The model under review builds one solid part; all positions refer to its coordinate system, in mm. Face numbers are marked on the shaded views. A direction names the side the tool comes from. Round coordinates to 2 decimals unless told otherwise and drop trailing zeros. Write each loop counter-clockwise with the first axis right and the second up, starting at its lowest first coordinate (ties: lowest second). Pieces come first, ordered by that corner, then holes. Notation, with made-up numbers: M -22.75,88 L 7.25,88 A31 ccw 7.25,117 Z; hole C 40,41.5 d6. An arc over 180 degrees is marked long. Write item = value, one per line. Start each with the question number.
Item 1: To check wall thickness, follow line 1 along Y through (x, z) = (19, 0.25); line 2 along Z through (x, y) = (-4, -1.5); line 3 along Y through (x, z) = (-6, -0.25). State the ranges of each line that lie inside material, in increasing order.
Item 2: Take a section at D-D, the plane y = -0.5. Give the boundary of the cut face in (x, z), plus the area to 3 significant figures.
Item 3: Take a section at C-C, the plane x = -2.5. Give the boundary of the cut face in (y, z).
Item 4: Take a section at A-A, the plane x = 43. Give the boundary of the cut face in (y, z).
Item 5: For pin 1 Ø2.5 at (y, z) = (-0.5, -1.5) entering from -X; pin 2 Ø3 at (y, z) = (0, -2) entering from +X; pin 3 Ø6 at (x, y) = (39.5, 0) entering from -Z; pin 4 Ø1.5 at (x, z) = (33, -0.5) entering from -Y, all flat-tipped, find the tip position at first contact; note any pin that passes through.
Item 6: Tool access review of the marked faces 1, 2 and 3: name each direction out of +Z, -Z, +X, -X, +Y, -Y from which nothing blocks a thin tool from reaching the whole face with its end or side.
Item 7: Take a section at B-B, the plane z = -1. Give the boundary of the cut face in (x, y).
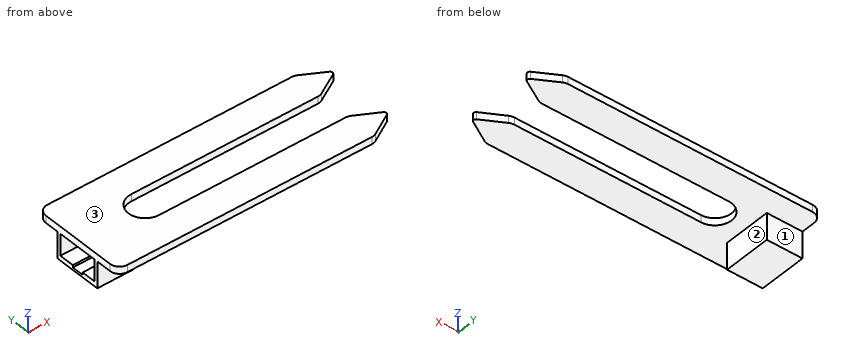
Autodesk Inventor part; units mm, degrees
ref_plane "YZ Plane" through (0, 0, 0) normal (1, 0, 0) x (0, 1, 0)
ref_plane "XZ Plane" through (0, 0, 0) normal (0, 1, 0) x (-1, 0, 0)
ref_plane "XY Plane" through (0, 0, 0) normal (0, 0, 1) x (1, 0, 0)
sketch "Sketch1" plane through (0, 0, 0) normal (0, 0, 1) x (1, 0, 0)
  line L0 (-9.4004, -0.0645) -> (24.8301, -0.0645)
  line L1 (-8.5062, -0.0645) -> (-8.5062, 8.0815)
  line L2 (-6.5062, 10.0815) -> (45.2045, 10.0815)
  line L3 (5.7396, 3.4575) -> (45.196, 3.4575)
  line L4 (-8.5062, -0.0645) -> (-8.5062, -8.2105)
  line L5 (-6.5062, -10.2105) -> (45.2045, -10.2105)
  line L6 (5.7396, -3.5865) -> (45.196, -3.5865)
  line L7 (50.7891, 7.186) -> (46.1991, 9.8167)
  line L8 (50.7862, 6.3168) -> (46.1793, 3.7159)
  line L9 (50.7891, -7.315) -> (46.1991, -9.9457)
  line L10 (50.7862, -6.4458) -> (46.1793, -3.8449)
  arc A0 (5.7396, 3.4575) -> (5.7396, -3.5865) centre (5.7054, -0.0645) ccw
  arc A1 (-6.5062, 10.0815) -> (-8.5062, 8.0815) centre (-6.5062, 8.0815) ccw
  arc A2 (-8.5062, -8.2105) -> (-6.5062, -10.2105) centre (-6.5062, -8.2105) ccw
  arc A3 (46.1991, 9.8167) -> (45.2045, 10.0815) centre (45.2045, 8.0815) ccw
  arc A4 (45.196, 3.4575) -> (46.1793, 3.7159) centre (45.196, 5.4575) ccw
  arc A5 (50.7862, 6.3168) -> (50.7891, 7.186) centre (50.5404, 6.7522) ccw
  line L11 (50.7891, -7.315) -> (46.1991, -9.9457)
  line L12 (50.7862, -6.4458) -> (46.1793, -3.8449)
  arc A6 (45.2045, -10.2105) -> (46.1991, -9.9457) centre (45.2045, -8.2105) ccw
  arc A7 (46.1793, -3.8449) -> (45.196, -3.5865) centre (45.196, -5.5865) ccw
  arc A8 (50.7891, -7.315) -> (50.7862, -6.4458) centre (50.5404, -6.8812) ccw
  line L13 (5.7396, 3.4575) -> (5.7396, 10.0815)
  line L14 (5.7396, -3.5865) -> (5.7396, -10.2105)
  point P0 (0, 0)
  point P1 (51.4938, 10.0604)
  point P2 (51.4938, -10.1894)
  dimension "d7" = 6.624
  dimension "d11" = 2
  dimension "d12" = 2
  dimension "d13" = 0.5
extrude "Extrusion1" add sketch "Sketch1" along normal blind 1.5 contours L13 L2 A3 L7 A5 L8 A4 L3 | L6 A7 L10 A8 L9 A6 L5 L14
extrude "Extrusion2" add sketch "Sketch1" along normal blind 1.5 contours L1 A1 L2 L13 A0 L0 | L0 A0 L14 L5 A2 L4
split_face "Split1"
sketch "Sketch2" plane through (-8.5062, -8.2105, 0) normal (0, 0, -1) x (-1, 0, 0)
  line L0 (0, 16.292) -> (0, 0)
  line L1 (0, 13.3304) -> (-7.5479, 13.3304)
  line L2 (-7.5479, 13.3304) -> (-7.5479, 3.2425)
  line L3 (-7.5479, 3.2425) -> (0, 3.2425)
  line L4 (0, 3.2425) -> (0, 13.3304)
  line L5 (-8.5062, 8.2105) -> (18.1258, 8.2105)
  point P0 (0, 3.2425)
  dimension "d16" = 7.5479
  dimension "d17" = 10.0879
  dimension "d18" = 4.968
extrude "Extrusion3" add sketch "Sketch2" along normal blind 5.6
sketch "Sketch4" plane through (-8.5062, -8.2105, 1.5) normal (-1, 0, 0) x (0, 0, 1)
  line L0 (-1.5, 11.668) -> (-1.5, 18.292)
  line L1 (-6.093, 3.9575) -> (-1.5, 3.9575)
  line L2 (-1.5, 3.9575) -> (-1.5, 12.6111)
  line L3 (-1.5, 12.6111) -> (-6.093, 12.6111)
  line L4 (-7.1, 3.2425) -> (-7.1, 13.3304)
  line L5 (-1.5, 3.2425) -> (-7.1, 3.2425)
  line L6 (-1.5, 13.3304) -> (-7.1, 13.3304)
  line L7 (-1.5, 8.2105) -> (-9.0756, 8.2105)
  line L8 (-6.093, 6.97) -> (-6.5947, 6.97)
  line L9 (-6.5947, 6.97) -> (-6.5947, 8.2105)
  line L10 (-6.093, 9.4509) -> (-6.5947, 9.4509)
  line L11 (-6.5947, 9.4509) -> (-6.5947, 8.2105)
  line L12 (-6.093, 12.6111) -> (-6.093, 9.4509)
  line L13 (-6.093, 6.97) -> (-6.093, 3.9575)
  dimension "d22" = 0.715
  dimension "d23" = 0.7192
extrude "Extrusion4" cut sketch "Sketch4" against normal blind 7.4 contours L2 L7 L11 L10 L12 L3 L0 | L2 L1 L13 L8 L9 L7
properties part number "sensorhumedad" material "Brass, Soft Yellow"
Response values:
q1.line_1 = -10.21 to -3.59, 3.46 to 10.08
q1.line_2 = -5.6 to -4.59, 0 to 1.5
q1.line_3 = -4.97 to -4.25, 4.4 to 5.12
q2.outline = M -8.51,-5.6 L -0.96,-5.6 L -0.96,0 L 2.21,0 L 2.21,1.5 L -8.51,1.5 L -8.51,0 L -1.11,0 L -1.11,-5.09 L -8.51,-5.09 Z
q2.area = 20.6 mm2
q3.outline = M -10.21,0 L -4.97,0 L -4.97,-5.6 L 5.12,-5.6 L 5.12,0 L 10.08,0 L 10.08,1.5 L -10.21,1.5 Z; hole M -4.25,-4.59 L -1.24,-4.59 L -1.24,-5.09 L 1.24,-5.09 L 1.24,-4.59 L 4.4,-4.59 L 4.4,0 L -4.25,0 Z
q4.outline = M -10.21,0 L -3.59,0 L -3.59,1.5 L -10.21,1.5 Z; M 3.46,0 L 10.08,0 L 10.08,1.5 L 3.46,1.5 Z
q5.pin_1 = -1.11
q5.pin_2 = -0.96
q5.pin_3 = through
q5.pin_4 = -10.21
q6.face_1 = -Z, +X, -X, +Y
q6.face_2 = -Z, +X, +Y, -Y
q6.face_3 = +Z, +X, -X, +Y, -Y
q7.outline = M -8.51,-4.97 L -0.96,-4.97 L -0.96,5.12 L -8.51,5.12 L -8.51,4.4 L -1.11,4.4 L -1.11,-4.25 L -8.51,-4.25 Z
